Read the model definition and answer for the solid it produces. Units are mm, in the model's axes. Face numbers are marked on the shaded views. Coordinates: 2 decimals unless noted, no trailing zeros. Order: outer loops, then holes, each group sorted by start corner. A loop starts at its lowest first (then second) coordinate and runs counter-clockwise, first axis right, second up. Notation, with made-up numbers: M -31,60.5 L 11,60.5 A14 cw 11,69.5 Z; hole C 75,-17.5 d9. An arc over 180 degrees is marked long. Use a Markdown table: item, result. Add a question column.
1) Find section A-A on z = -4. Write down the section's boundary in (x, y), plus the area to 3 significant figures.
2) Find section B-B on x = -7. Write down the section's boundary in (y, z).
3) Find the intervals of material crossed by probe 1 along X at (y, z) = (3, -2.75); probe 2 along X at (y, z) = (5, -6); probe 3 along X at (y, z) = (6.75, -5), in increasing order. Write a range as [from, to].
4) Find section D-D on z = -2.5. Write down the section's boundary in (x, y).
5) The mould has two halves that part along Y. Classify the marked faces 1, 2 and 3: released by +Y, released by -Y, zero draft, split by the parting line, or undercut.
6) Find section C-C on y = 3.5. Write down the section's boundary in (x, z).
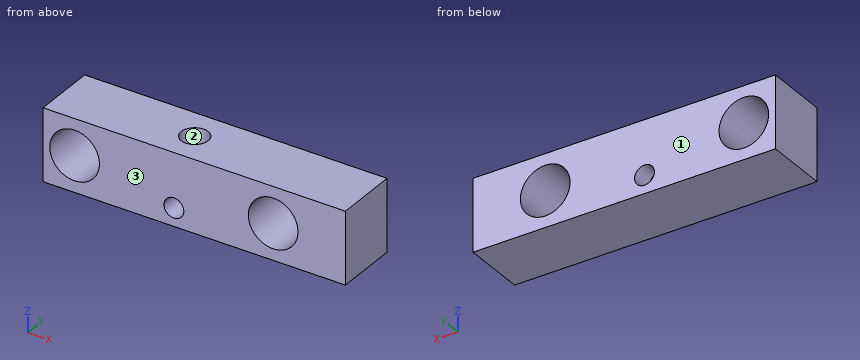
from build123d import *

# Parameters (mm, degrees)
SKETCH_1_W          = 38
SKETCH_1_H          = 8
SKETCH_1_R          = 2.75
SKETCH_1_R_2        = 1.1
EXTRUDE_1_DEPTH     = 7
SKETCH_2_W          = 4.5
SKETCH_2_H          = 7
CUT_EXTRUDE_1_DEPTH = 27.617640313
SKETCH_4_R          = 1.5
CUT_EXTRUDE_2_DEPTH = 6


with BuildPart() as part:
    # 草图1 → 凸台-拉伸1 (new body)
    with BuildSketch(Plane(origin=(0, 0, 0), x_dir=(1, 0, 0), z_dir=(0, 1, 0))):
        with Locations((5.402843602, 4.239336493)):
            Rectangle(SKETCH_1_W, SKETCH_1_H)
        with Locations(Location((-5.597156398, 4.239336493, 0), (0, 0, 270))):
            Circle(SKETCH_1_R, mode=Mode.SUBTRACT)
        with Locations(Location((16.402843602, 4.239336493, 0), (0, 0, 270))):
            Circle(SKETCH_1_R, mode=Mode.SUBTRACT)
        with Locations(Location((5.402843602, 6.239336493, 0), (0, 0, 270))):
            Circle(SKETCH_1_R_2, mode=Mode.SUBTRACT)
    extrude(amount=EXTRUDE_1_DEPTH)

    # 草图2 → 切除-拉伸1 (cut, through all)
    with BuildSketch(Plane.XY.offset(-0.239336493)):
        with Locations((-11.347156398, 3.5)):
            Rectangle(SKETCH_2_W, SKETCH_2_H)
    extrude(amount=-CUT_EXTRUDE_1_DEPTH, mode=Mode.SUBTRACT)

    # 草图4 → 切除-拉伸2 (cut)
    with BuildSketch(Plane.XY.offset(-0.239336493)):
        with Locations((5.402843602, 3.5)):
            Circle(SKETCH_4_R)
    extrude(amount=-CUT_EXTRUDE_2_DEPTH, mode=Mode.SUBTRACT)


solid = part.part
Check result:
| question | item | result |
|---|---|---|
| 1 | outline | M -9.1,0 L -8.34,0 L -8.34,7 L -9.1,7 Z; M -2.86,0 L 13.66,0 L 13.66,7 L -2.86,7 Z; M 19.14,0 L 24.4,0 L 24.4,7 L 19.14,7 Z; hole C 5.4,3.5 d3 |
| 1 | area | 151 mm2 |
| 2 | outline | M 0,-8.24 L 7,-8.24 L 7,-6.6 L 0,-6.6 Z; M 0,-1.87 L 7,-1.87 L 7,-0.24 L 0,-0.24 Z |
| 3 | probe 1 | x = [-9.1, -7.91], [-3.29, 3.99], [6.82, 14.09], [18.71, 24.4] |
| 3 | probe 2 | x = [-9.1, -7.71], [-3.48, 4.33], [6.48, 14.29], [18.52, 24.4] |
| 3 | probe 3 | x = [-9.1, -8.24], [-2.95, 13.76], [19.05, 24.4] |
| 4 | outline | M -9.1,0 L -7.73,0 L -7.73,7 L -9.1,7 Z; M -3.47,0 L 14.27,0 L 14.27,7 L -3.47,7 Z; M 18.53,0 L 24.4,0 L 24.4,7 L 18.53,7 Z; hole C 5.4,3.5 d3 |
| 5 | face 1 | released by +Y |
| 5 | face 2 | undercut |
| 5 | face 3 | released by -Y |
| 6 | outline | M -9.1,-8.24 L 24.4,-8.24 L 24.4,-0.24 L 6.9,-0.24 L 6.9,-6.24 L 6.5,-6.24 A1.1 cw 4.3,-6.24 L 3.9,-6.24 L 3.9,-0.24 L -9.1,-0.24 Z; hole C -5.6,-4.24 d5.5; hole C 16.4,-4.24 d5.5 |
